from build123d import *

# Parameters (mm, degrees)
CROQUIS1_W              = 150.4
CROQUIS1_H              = 44
SALIENTE_EXTRUIR1_DEPTH = 1.2
CROQUIS2_W              = 44
CROQUIS2_H              = 1.2
SALIENTE_EXTRUIR2_DEPTH = 4
CHAFL_N1_SIZE           = 0.4
CHAFL_N2_SIZE           = 1


with BuildPart() as part:
    # Croquis1 → Saliente-Extruir1 (new body)
    with BuildSketch(Plane(origin=(0, 0, 0), x_dir=(0, 1, 0), z_dir=(0, 0, 1))):
        Rectangle(CROQUIS1_W, CROQUIS1_H)
    extrude(amount=SALIENTE_EXTRUIR1_DEPTH)

    # Croquis2 → Saliente-Extruir2 (add)
    with BuildSketch(Plane.XY.offset(1.2)):
        with Locations((0, 74.6)):
            Rectangle(CROQUIS2_W, CROQUIS2_H)
        with Locations((0, -74.6)):
            Rectangle(CROQUIS2_W, CROQUIS2_H)
        with Locations((0, -62.9)):
            Rectangle(CROQUIS2_W, CROQUIS2_H)
        with Locations((0, 62.9)):
            Rectangle(CROQUIS2_W, CROQUIS2_H)
    extrude(amount=SALIENTE_EXTRUIR2_DEPTH)

    # Chaflán1
    chafl_n1_edges = [part.edges().sort_by_distance(p)[0] for p in [
        (0, 74, 1.2),
        (0, -74, 1.2),
        (0, -63.5, 1.2),
        (0, -62.3, 1.2),
        (0, 62.3, 1.2),
        (0, 63.5, 1.2),
    ]]
    chamfer(chafl_n1_edges, length=CHAFL_N1_SIZE)

    # Chaflán2
    chafl_n2_edges = [part.edges().sort_by_distance(p)[0] for p in [
        (0, -75.2, 0),
        (0, 75.2, 0),
    ]]
    chamfer(chafl_n2_edges, length=CHAFL_N2_SIZE)


solid = part.part
For this review, take the finished solid that the model builds, in its own axes (mm). A direction names the side the tool comes from. Coordinates: 2 decimals unless noted, no trailing zeros. Order: outer loops, then holes, each group sorted by start corner. A loop starts at its lowest first (then second) coordinate and runs counter-clockwise, first axis right, second up. Notation, with made-up numbers: (-37, -27.5) - (-3, -27.5) arc R15 cw to (-3, -3.5) - close; hole circle Ø2 at (5, 54.25). An arc over 180 degrees is marked (long way). Answer as CSV lines item,"result". Start each with the question number.
1) Machinability: for faces 1 (the flat face through (0, -75.2, 3)), 2 (the flat face through (0, 62.3, 3)), which of the approach directions +Z, -Z, +X, -X, +Y, -Y give a long, thin tool a straight path to every point of the face, cutting with its end or side? Answer none if there is none.
2) To check wall thickness, follow line 1 along Y through (x, z) = (-16.5, 3.25); line 2 along Y through (x, z) = (-13, 1.35); line 3 along Z through (x, y) = (16, -51). State the ranges of each line that lie inside material, in increasing order. Write a range as [from, to].
3) Add section C-C (y = 3). State the section outline as (x, z) points.
4) Add section A-A (z = 2.85). State the section outline as (x, y) points, then the cut area to 3 significant figures.
5) Draft analysis for pull direction Y (two halves, no side actions). For faces 3 (the flat face through (0, -69, 1.2)), 4 (the flat face through (0, 75.2, 3)), 5 (the flat face through (22, -0.4, 0.5)), state which applies: +Y half, -Y half, draft (parallel to the pull), parting line (faces both ways), or undercut.
6) Insertion check: P1, Ø5, axis at x = 10.5, y = 70.5, coming from the +Z side. The pin has a flat end and moves straight along its axis. Give the tip position at first contact, or say it passes through.
7) Add section B-B (x = -1). State the section outline as (y, z) points, then the cut area to 3 significant figures.
Result:
1,face 1,"+Z, -Z, +X, -X, -Y"
1,face 2,"+Z, +X, -X"
2,line 1,"[-75.2, -74], [-63.5, -62.3], [62.3, 63.5], [74, 75.2]"
2,line 2,"[-75.2, -73.75], [-63.75, -62.05], [62.05, 63.75], [73.75, 75.2]"
2,line 3,"[0, 1.2]"
3,outline,"(-22, 0) - (22, 0) - (22, 1.2) - (-22, 1.2) - close"
4,outline,"(-22, -75.2) - (22, -75.2) - (22, -74) - (-22, -74) - close; (-22, -63.5) - (22, -63.5) - (22, -62.3) - (-22, -62.3) - close; (-22, 62.3) - (22, 62.3) - (22, 63.5) - (-22, 63.5) - close; (-22, 74) - (22, 74) - (22, 75.2) - (-22, 75.2) - close"
4,area,"211 mm^2"
5,face 3,"undercut"
5,face 4,"+Y half"
5,face 5,"draft"
6,P1,"z = 1.2"
7,outline,"(-75.2, 1) - (-74.2, 0) - (74.2, 0) - (75.2, 1) - (75.2, 5.2) - (74, 5.2) - (74, 1.6) - (73.6, 1.2) - (63.9, 1.2) - (63.5, 1.6) - (63.5, 5.2) - (62.3, 5.2) - (62.3, 1.6) - (61.9, 1.2) - (-61.9, 1.2) - (-62.3, 1.6) - (-62.3, 5.2) - (-63.5, 5.2) - (-63.5, 1.6) - (-63.9, 1.2) - (-73.6, 1.2) - (-74, 1.6) - (-74, 5.2) - (-75.2, 5.2) - close"
7,area,"199 mm^2"
